```python
from build123d import *

# Parameters (mm, degrees)
F0_R     = 1.820251
F1_DEPTH = 3


with BuildPart() as f1:
    # F0 (on Top) → F1 (new body)
    with BuildSketch(Plane.XY):
        with BuildLine():
            ThreePointArc((7.178103, 13.170985), (5.931993, 13.777208), (4.635255, 14.265848))
            ThreePointArc((4.635255, 14.265848), (3.298957, 14.632733), (1.934503, 14.874734))
            ThreePointArc((1.934503, 14.874734), (0, 21.67554), (-1.934503, 14.874734))
            ThreePointArc((-1.934503, 14.874734), (-3.298957, 14.632733), (-4.635255, 14.265848))
            ThreePointArc((-4.635255, 14.265848), (-5.931993, 13.777208), (-7.178103, 13.170985))
            ThreePointArc((-7.178103, 13.170985), (-12.740563, 17.53588), (-10.308195, 10.89684))
            ThreePointArc((-10.308195, 10.89684), (-11.269817, 9.899052), (-12.135255, 8.816779))
            ThreePointArc((-12.135255, 8.816779), (-12.897123, 7.659258), (-13.548918, 6.436367))
            ThreePointArc((-13.548918, 6.436367), (-20.614663, 6.69811), (-14.744507, 2.756724))
            ThreePointArc((-14.744507, 2.756724), (-14.93599, 1.384269), (-15, 0))
            ThreePointArc((-15, 0), (-14.93599, -1.384269), (-14.744507, -2.756724))
            ThreePointArc((-14.744507, -2.756724), (-20.614663, -6.69811), (-13.548918, -6.436367))
            ThreePointArc((-13.548918, -6.436367), (-12.897123, -7.659258), (-12.135255, -8.816779))
            ThreePointArc((-12.135255, -8.816779), (-11.269817, -9.899052), (-10.308195, -10.89684))
            ThreePointArc((-10.308195, -10.89684), (-12.740563, -17.53588), (-7.178103, -13.170985))
            ThreePointArc((-7.178103, -13.170985), (-5.931993, -13.777208), (-4.635255, -14.265848))
            ThreePointArc((-4.635255, -14.265848), (-3.298957, -14.632733), (-1.934503, -14.874734))
            ThreePointArc((-1.934503, -14.874734), (0, -21.67554), (1.934503, -14.874734))
            ThreePointArc((1.934503, -14.874734), (3.298957, -14.632733), (4.635255, -14.265848))
            ThreePointArc((4.635255, -14.265848), (5.931993, -13.777208), (7.178103, -13.170985))
            ThreePointArc((7.178103, -13.170985), (12.740563, -17.53588), (10.308195, -10.89684))
            ThreePointArc((10.308195, -10.89684), (11.269817, -9.899052), (12.135255, -8.816779))
            ThreePointArc((12.135255, -8.816779), (12.897123, -7.659258), (13.548918, -6.436367))
            ThreePointArc((13.548918, -6.436367), (20.614663, -6.69811), (14.744507, -2.756724))
            ThreePointArc((14.744507, -2.756724), (14.93599, -1.384269), (15, 0))
            ThreePointArc((15, 0), (14.93599, 1.384269), (14.744507, 2.756724))
            ThreePointArc((14.744507, 2.756724), (20.614663, 6.69811), (13.548918, 6.436367))
            ThreePointArc((13.548918, 6.436367), (12.897123, 7.659258), (12.135255, 8.816779))
            ThreePointArc((12.135255, 8.816779), (11.269817, 9.899052), (10.308195, 10.89684))
            ThreePointArc((10.308195, 10.89684), (12.740563, 17.53588), (7.178103, 13.170985))
        make_face()
        with Locations((-10.580135, -14.562306)):
            Circle(F0_R, mode=Mode.SUBTRACT)
        with Locations((-17.119017, -5.562306)):
            Circle(F0_R, mode=Mode.SUBTRACT)
        with Locations((0, -18)):
            Circle(F0_R, mode=Mode.SUBTRACT)
        with Locations((10.580135, -14.562306)):
            Circle(F0_R, mode=Mode.SUBTRACT)
        with Locations((17.119017, -5.562306)):
            Circle(F0_R, mode=Mode.SUBTRACT)
        with Locations((-17.119017, 5.562306)):
            Circle(F0_R, mode=Mode.SUBTRACT)
        with Locations((-10.580135, 14.562306)):
            Circle(F0_R, mode=Mode.SUBTRACT)
        with BuildLine():
            ThreePointArc((0, 11), (1.720779, 10.864572), (3.399187, 10.461622))
            ThreePointArc((3.399187, 10.461622), (6.465638, 8.899187), (8.899187, 6.465638))
            ThreePointArc((8.899187, 6.465638), (10.461622, 3.399187), (11, 0))
            ThreePointArc((11, 0), (10.461622, -3.399187), (8.899187, -6.465638))
            ThreePointArc((8.899187, -6.465638), (6.465638, -8.899187), (3.399187, -10.461622))
            ThreePointArc((3.399187, -10.461622), (0, -11), (-3.399187, -10.461622))
            ThreePointArc((-3.399187, -10.461622), (-6.465638, -8.899187), (-8.899187, -6.465638))
            ThreePointArc((-8.899187, -6.465638), (-10.461622, -3.399187), (-11, 0))
            ThreePointArc((-11, 0), (-10.461622, 3.399187), (-8.899187, 6.465638))
            ThreePointArc((-8.899187, 6.465638), (-6.465638, 8.899187), (-3.399187, 10.461622))
            ThreePointArc((-3.399187, 10.461622), (-1.720779, 10.864572), (0, 11))
        make_face(mode=Mode.SUBTRACT)
        with Locations((17.119017, 5.562306)):
            Circle(F0_R, mode=Mode.SUBTRACT)
        with BuildLine():
            ThreePointArc((0, 16.179749), (-1.287112, 19.287112), (1.820251, 18))
            ThreePointArc((1.820251, 18), (1.287112, 16.712888), (0, 16.179749))
        make_face(mode=Mode.SUBTRACT)
        with Locations((10.580135, 14.562306)):
            Circle(F0_R, mode=Mode.SUBTRACT)
    extrude(amount=F1_DEPTH)


solid = f1.part
```
Design review of the part built by this model. Coordinates are the model's own, in mm. Give positions to 0.01 mm unless a question says otherwise; leave off trailing zeros. Order: outer loops, then holes, each group sorted by start corner. A loop starts at its lowest first (then second) coordinate and runs counter-clockwise, first axis right, second up. Notation, with made-up numbers: (6, -12.5) - (47, -12.5) arc R17 ccw to (47, -2.5) - close; hole circle Ø11 at (-18, 5). An arc over 180 degrees is marked (long way). Use a Markdown table: item, result. Add a question column.
(1) Add section A-A on x = 17. Give the boundary of the cut face in (y, z), then the cut area to 3 significant figures.
(2) Add section B-B on y = -0.5. Give the boundary of the cut face in (x, z), then the cut area to 3 significant figures.
(3) Add section C-C on y = 17. Give the boundary of the cut face in (x, z), then the cut area to 3 significant figures.
(4) Clearance check with a flat-ended pin moving along its axis: P1, Ø3, axis at x = -17.12, y = -5.56, coming from the +Z side. State where the tip first meets the part, or that it passes through.
(5) Wall thickness on probe 1 along Y at (x, z) = (0, 2.35); probe 2 along Y at (x, z) = (13, 1.45); probe 3 along X at (y, z) = (-7, 1.35): over which ranges is each line inside the solid? List them lowest first. Write a range as [from, to].
(6) Add section D-D on z = 2.5. Give the number of separate pieces and of enclosed holes in the cut face, then the cut area to 3 significant figures.
Report:
| question | item | result |
|---|---|---|
| 1 | outline | (-9.24, 0) - (-7.38, 0) - (-7.38, 3) - (-9.24, 3) - close; (-3.75, 0) - (-1.89, 0) - (-1.89, 3) - (-3.75, 3) - close; (1.89, 0) - (3.75, 0) - (3.75, 3) - (1.89, 3) - close; (7.38, 0) - (9.24, 0) - (9.24, 3) - (7.38, 3) - close |
| 1 | area | 22.3 mm² |
| 2 | outline | (-14.99, 0) - (-10.99, 0) - (-10.99, 3) - (-14.99, 3) - close; (10.99, 0) - (14.99, 0) - (14.99, 3) - (10.99, 3) - close |
| 2 | area | 24.0 mm² |
| 3 | outline | (-13.33, 0) - (-7.83, 0) - (-7.83, 3) - (-13.33, 3) - close; (-3.54, 0) - (-1.52, 0) - (-1.52, 3) - (-3.54, 3) - close; (1.52, 0) - (3.54, 0) - (3.54, 3) - (1.52, 3) - close; (7.83, 0) - (13.33, 0) - (13.33, 3) - (7.83, 3) - close |
| 3 | area | 45.1 mm² |
| 4 | P1 | passes through |
| 5 | probe 1 | y = [-21.68, -19.82], [-16.18, -11], [11, 16.18], [19.82, 21.68] |
| 5 | probe 2 | y = [-17.33, -11.8], [-7.48, 7.48], [11.8, 17.33] |
| 5 | probe 3 | x = [-20.5, -18.24], [-16, -13.74], [-13.27, -8.49], [8.49, 13.27], [13.74, 16], [18.24, 20.5] |
| 6 | separate pieces | 1 |
| 6 | enclosed holes | 11 |
| 6 | area | 629 mm² |
